For this review, take the finished solid that the model builds, in its own axes (mm). A direction names the side the tool comes from. Round coordinates to 2 decimals unless told otherwise and drop trailing zeros. Order: outer loops, then holes, each group sorted by start corner. A loop starts at its lowest first (then second) coordinate and runs counter-clockwise, first axis right, second up. Notation, with made-up numbers: (-27.75, 78) - (9.25, 78) arc R28 cw to (9.25, 112) - close; hole circle Ø2 at (24, 53). An arc over 180 degrees is marked (long way). Write each question's results on one line, items separated by ' | '. Start each with the question number.
(1) Take a section at B-B, the plane z = 5. Give the boundary of the cut face in (x, y).
(2) For L1, parallel to X at y = 27.5, z = 4.9; L2, parallel to Y at x = 53, z = 2.75; L3, parallel to X at y = 35.25, z = 3.2, list the stretches that pass through material, from the lowest coordinate up. Write a range as from..to.
(3) For faces 1 (the flat face through (53, 26.6, 5)), 2 (the cylindrical face through (52.3, 28.1, 4.1)), list the 3-axis set-ups (+Z, -Z, +X, -X, +Y, -Y) from which the entire face can be reached by the end or side of a thin tool; tool diameter is ignored.
(4) Take a section at A-A, the plane x = 53.5. Give the boundary of the cut face in (y, z).
(5) Take a section at D-D, the plane z = 2.7. Give the boundary of the cut face in (x, y), plus the area to 3 significant figures.
(6) Take a section at C-C, the plane y = 33. Give the boundary of the cut face in (x, z), plus the area to 3 significant figures.
```python
from build123d import *

# Parameters (mm, degrees)
CYLINDER012_R     = 2.7
CYLINDER012_DEPTH = 8
CYLINDER008_R     = 1.5
CYLINDER008_DEPTH = 11


with BuildPart() as cylinder012:
    # Cylinder012 → Cylinder012 (new body)
    with BuildSketch(Plane(origin=(53.5, 37.6, 5), x_dir=(1, 0, 0), z_dir=(0, -1, 0))):
        Circle(CYLINDER012_R)
    extrude(amount=CYLINDER012_DEPTH)


with BuildPart() as fusion016:
    # Cylinder008 → Cylinder008 (new body)
    with BuildSketch(Plane(origin=(53.5, 37.6, 5), x_dir=(1, 0, 0), z_dir=(0, -1, 0))):
        Circle(CYLINDER008_R)
    extrude(amount=CYLINDER008_DEPTH)

    # Fusion016: union Cylinder012
    add(cylinder012.part)


solid = fusion016.part
```
Results below:
1) outline: (50.8, 29.6) - (52, 29.6) - (52, 26.6) - (55, 26.6) - (55, 29.6) - (56.2, 29.6) - (56.2, 37.6) - (50.8, 37.6) - close
2) L1: x = 52..55 | L2: y = 29.6..37.6 | L3: x = 51.49..55.51
3) face 1: +Z, -Z, +X, -X, -Y | face 2: -Y
4) outline: (26.6, 3.5) - (29.6, 3.5) - (29.6, 2.3) - (37.6, 2.3) - (37.6, 7.7) - (29.6, 7.7) - (29.6, 6.5) - (26.6, 6.5) - close
5) outline: (52.09, 29.6) - (54.91, 29.6) - (54.91, 37.6) - (52.09, 37.6) - close | area: 22.6 mm^2
6) outline: circle Ø5.4 at (53.5, 5) | area: 22.9 mm^2
